Could you check a few things on this model? Use its own coordinates, in mm. Face numbers are marked on the shaded views. A direction names the side the tool comes from. Round coordinates to 2 decimals unless told otherwise and drop trailing zeros. Loops run counter-clockwise (first coordinate to the right, second up) from the corner with the lowest first, then second, coordinate; pieces in that order, holes last.
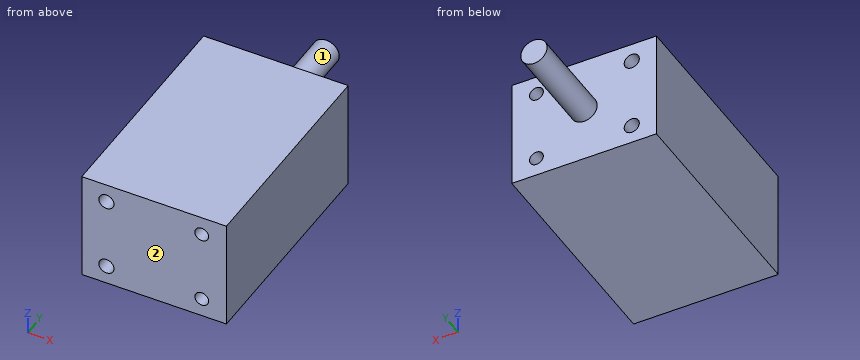
from build123d import *

# Parameters (mm, degrees)
F_01_HOUSING_PROFILE_W      = 55
F_01_HOUSING_PROFILE_H      = 42
F_01_HOUSING_PROFILE_R      = 2.877277304
F_01_HOUSING_PROFILE_R_2    = 2.627218626
F_01_HOUSING_BLOCK_DEPTH    = 85
F_03_OUTPUT_SHAFT_PROFILE_R = 5
F_03_OUTPUT_SHAFT_DEPTH     = 120


with BuildPart() as part:
    # 01_Housing_Profile → 01_Housing_Block (new body)
    with BuildSketch(Plane(origin=(0, 0, 0), x_dir=(1, 0, 0), z_dir=(0, 1, 0))):
        Rectangle(F_01_HOUSING_PROFILE_W, F_01_HOUSING_PROFILE_H)
        with Locations(Location((-18.122781374, -13.839214867, 0), (0, 0, 270))):
            Circle(F_01_HOUSING_PROFILE_R, mode=Mode.SUBTRACT)
        with Locations(Location((18.122781374, -13.839214867, 0), (0, 0, 270))):
            Circle(F_01_HOUSING_PROFILE_R_2, mode=Mode.SUBTRACT)
        with Locations(Location((-18.122781374, 13.839214867, 0), (0, 0, 270))):
            Circle(F_01_HOUSING_PROFILE_R, mode=Mode.SUBTRACT)
        with Locations(Location((18.122781374, 13.839214867, 0), (0, 0, 270))):
            Circle(F_01_HOUSING_PROFILE_R_2, mode=Mode.SUBTRACT)
    extrude(amount=F_01_HOUSING_BLOCK_DEPTH)

    # 03_Output_Shaft_Profile → 03_Output_Shaft (add)
    with BuildSketch(Plane(origin=(0, 0, 0), x_dir=(1, 0, 0), z_dir=(0, 1, 0))):
        with Locations(Location((0, 0, 0), (0, 0, 90))):
            Circle(F_03_OUTPUT_SHAFT_PROFILE_R)
    extrude(amount=F_03_OUTPUT_SHAFT_DEPTH)


solid = part.part
Item 1: If we section it at D-D, the plane z = 0: Please give me the cut outline in (x, y).
Results list:
outline: (-27.5, 0) - (27.5, 0) - (27.5, 85) - (5, 85) - (5, 120) - (-5, 120) - (-5, 85) - (-27.5, 85) - close
Item 2: If I drill on line 1 along Z through (x, y) = (18, 33.5); line 2 along X through (y, z) = (47, -12.5); line 3 along Z through (x, y) = (-20, 27), over which ranges is the centre line in solid material (lowest first)?
Results list:
line 1: z = -21 to -16.46, -11.21 to 11.21, 16.46 to 21
line 2: x = -27.5 to -20.67, -15.58 to 15.86, 20.38 to 27.5
line 3: z = -21 to -16.02, -11.66 to 11.66, 16.02 to 21
Item 3: If we section it at A-A, the plane z = 12.5: Please give me the cut outline in (x, y).
Results list:
outline: (-27.5, 0) - (-20.67, 0) - (-20.67, 85) - (-27.5, 85) - close; (-15.58, 0) - (15.86, 0) - (15.86, 85) - (-15.58, 85) - close; (20.38, 0) - (27.5, 0) - (27.5, 85) - (20.38, 85) - close
Item 4: If we section it at C-C, the plane x = 0: Please give me the cut outline in (y, z), then the cut area to 3 significant figures.
Results list:
outline: (0, -21) - (85, -21) - (85, -5) - (120, -5) - (120, 5) - (85, 5) - (85, 21) - (0, 21) - close
area: 3,920 mm2
Item 5: If we section it at B-B, the plane y = 30.5: Please give me the cut outline in (x, z).
Results list:
outline: (-27.5, -21) - (27.5, -21) - (27.5, 21) - (-27.5, 21) - close; hole circle Ø5.75 at (-18.12, -13.84); hole circle Ø5.75 at (-18.12, 13.84); hole circle Ø5.25 at (18.12, -13.84); hole circle Ø5.25 at (18.12, 13.84)
Item 6: For the marked faces 1 and 2, which set-ups out of +Z, -Z, +X, -X, +Y, -Y let a thin tool reach every point of the face, with its end or its side?
Results list:
face 1: +Y
face 2: +Z, -Z, +X, -X, -Y
Item 7: Will these pins go through, and if not, where does the flat tip stop? pin 1 (9 mm diameter, centred on x = -18.12, z = 13.84, fed in from +Y); pin 2 (4.5 mm diameter, centred on x = 18.12, z = -13.84, fed in from -Y); pin 3 (1.5 mm diameter, centred on x = -4, y = 99.5, fed in from +Z); pin 4 (6 mm diameter, centred on x = 18.12, z = 13.84, fed in from -Y).
Results list:
pin 1: stops at y = 85
pin 2: passes through
pin 3: stops at z = 3.8
pin 4: stops at y = 0
